```python
from build123d import *

# Parameters (mm, degrees)
F0_W     = 101.6
F0_H     = 101.6
F1_DEPTH = 9.525
F2_W     = 88.9
F2_H     = 88.9
F3_DEPTH = 3.175
F5_DEPTH = 3.175
F6_R     = 4.7625
F6_R_2   = 12.7
F7_DEPTH = 6.351
F8_R     = 3.175
F9_DEPTH = 9.526


with BuildPart() as f1:
    # F0 (on Top) → F1 (new body)
    with BuildSketch(Plane.XY):
        with Locations((50.8, 50.8)):
            Rectangle(F0_W, F0_H)
    extrude(amount=F1_DEPTH)

    # F2 (on face) → F3 (cut)
    with BuildSketch(Plane.XY.offset(9.525)):
        with Locations((50.8, 50.8)):
            Rectangle(F2_W, F2_H)
    extrude(amount=-F3_DEPTH, mode=Mode.SUBTRACT)

    # F4 (on face) → F5 (cut)
    with BuildSketch(Plane.XY.offset(9.525)):
        with BuildLine():
            Line((6.35, 95.25), (2.8575, 95.25))
            ThreePointArc((2.8575, 95.25), (1.2474604822, 94.8567465215), (0, 93.7655463142))
            Line((0, 93.7655463142), (0, 89.7494536858))
            ThreePointArc((0, 89.7494536858), (1.2474604822, 88.6582534785), (2.8575, 88.265))
            ThreePointArc((2.8575, 88.265), (5.3270704333, 87.2420704333), (6.35, 84.7725))
            Line((6.35, 84.7725), (6.35, 95.25))
        make_face()
        with BuildLine():
            ThreePointArc((2.8575, 13.335), (1.2474604822, 12.9417465215), (0, 11.8505463142))
            Line((0, 11.8505463142), (0, 7.8344536858))
            ThreePointArc((0, 7.8344536858), (1.2474604822, 6.7432534785), (2.8575, 6.35))
            Line((2.8575, 6.35), (6.35, 6.35))
            Line((6.35, 6.35), (6.35, 16.8275))
            ThreePointArc((6.35, 16.8275), (5.3270704333, 14.3579295667), (2.8575, 13.335))
        make_face()
        with BuildLine():
            ThreePointArc((98.7425, 13.335), (96.2729295667, 14.3579295667), (95.25, 16.8275))
            Line((95.25, 16.8275), (95.25, 6.35))
            Line((95.25, 6.35), (98.7425, 6.35))
            ThreePointArc((98.7425, 6.35), (100.3525395178, 6.7432534785), (101.6, 7.8344536858))
            Line((101.6, 7.8344536858), (101.6, 11.8505463142))
            ThreePointArc((101.6, 11.8505463142), (100.3525395178, 12.9417465215), (98.7425, 13.335))
        make_face()
        with BuildLine():
            Line((98.7425, 95.25), (95.25, 95.25))
            Line((95.25, 95.25), (95.25, 84.7725))
            ThreePointArc((95.25, 84.7725), (96.2729295667, 87.2420704333), (98.7425, 88.265))
            ThreePointArc((98.7425, 88.265), (100.3525395178, 88.6582534785), (101.6, 89.7494536858))
            Line((101.6, 89.7494536858), (101.6, 93.7655463142))
            ThreePointArc((101.6, 93.7655463142), (100.3525395178, 94.8567465215), (98.7425, 95.25))
        make_face()
    extrude(amount=-F5_DEPTH, mode=Mode.SUBTRACT)

    # F6 (on face) → F7 (cut, through all)
    with BuildSketch(Plane.XY.offset(6.35)):
        with Locations((23.8592316368, 77.7407683632)):
            Circle(F6_R)
        with Locations((77.7407683632, 77.7407683632)):
            Circle(F6_R)
        with Locations((77.7407683632, 23.8592316368)):
            Circle(F6_R)
        with Locations((23.8592316368, 23.8592316368)):
            Circle(F6_R)
        with Locations((50.8, 50.8)):
            Circle(F6_R_2)
    extrude(amount=-F7_DEPTH, mode=Mode.SUBTRACT)

    # F8 (on face) → F9 (cut, through all)
    with BuildSketch(Plane.XY.offset(9.525)):
        with Locations((12.7, 12.7)):
            Circle(F8_R)
        with Locations((88.9, 88.9)):
            Circle(F8_R)
        with Locations((12.7, 88.9)):
            Circle(F8_R)
        with Locations((88.9, 12.7)):
            Circle(F8_R)
    extrude(amount=-F9_DEPTH, mode=Mode.SUBTRACT)


solid = f1.part
```
Work out the finished part from the listing and answer in its coordinate system (mm). A direction names the side the tool comes from. Round coordinates to 2 decimals unless told otherwise and drop trailing zeros. Loops run counter-clockwise (first coordinate to the right, second up) from the corner with the lowest first, then second, coordinate; pieces in that order, holes last.
(1) The mould has two halves that part along Y. Classify faces 1 (the flat face through (50, 3, 9.525)), 2 (the flat face through (50, 101.6, 5)), 3 (the flat face through (51, 95.25, 8)): pulls with the +Y half, pulls with the -Y half, needs draft (parallel to the pull), parting line crosses it, or undercut.
Computed values:
face 1: needs draft
face 2: pulls with the +Y half
face 3: undercut
(2) The part is cut by section B-B, the plane y = 55.5. Give the vertices of the cut face in (x, z) (3 decimals).
Computed values:
outline: (0, 0) - (39.002, 0) - (39.002, 6.35) - (6.35, 6.35) - (6.35, 9.525) - (0, 9.525) - close; (62.598, 0) - (101.6, 0) - (101.6, 9.525) - (95.25, 9.525) - (95.25, 6.35) - (62.598, 6.35) - close
(3) The part is cut by section A-A, the plane x = 88.9. Give the vertices of the cut face in (y, z) (3 decimals), and give its area (3 significant figures).
Computed values:
outline: (0, 0) - (9.525, 0) - (9.525, 6.35) - (6.35, 6.35) - (6.35, 9.525) - (0, 9.525) - close; (15.875, 0) - (85.725, 0) - (85.725, 6.35) - (15.875, 6.35) - close; (92.075, 0) - (101.6, 0) - (101.6, 9.525) - (95.25, 9.525) - (95.25, 6.35) - (92.075, 6.35) - close
area: 605 mm2
(4) The part is cut by section C-C, the plane x = 55. Give the vertices of the cut face in (y, z) (3 decimals), and give its area (3 significant figures).
Computed values:
outline: (0, 0) - (38.815, 0) - (38.815, 6.35) - (6.35, 6.35) - (6.35, 9.525) - (0, 9.525) - close; (62.785, 0) - (101.6, 0) - (101.6, 9.525) - (95.25, 9.525) - (95.25, 6.35) - (62.785, 6.35) - close
area: 533 mm2
(5) Each of these flat-tipped pins is pushed along its axis until it touches: P1, Ø10, axis at x = 88.9, y = 12.7, coming from the -Z side; P2, Ø11, axis at x = 77.74, y = 23.86, coming from the +Z side. Where does it stop, or does it pass through?
Computed values:
P1: stops at z = 0
P2: stops at z = 6.35
(6) The part is cut by section D-D, the plane y = 81. Give the vertices of the cut face in (x, z) (3 decimals).
Computed values:
outline: (0, 0) - (20.387, 0) - (20.387, 6.35) - (6.35, 6.35) - (6.35, 9.525) - (0, 9.525) - close; (27.332, 0) - (74.268, 0) - (74.268, 6.35) - (27.332, 6.35) - close; (81.213, 0) - (101.6, 0) - (101.6, 9.525) - (95.25, 9.525) - (95.25, 6.35) - (81.213, 6.35) - close
(7) Find the intervals of material crossed by L1, parallel to Y at x = 88.9, z = 5.25 (3 decimals); L2, parallel to Y at x = 24.5, z = 0.5; L3, parallel to X at y = 82, z = 3.75, in increasing order.
Computed values:
L1: y = 0 to 9.525, 15.875 to 85.725, 92.075 to 101.6
L2: y = 0 to 19.14, 28.58 to 73.02, 82.46 to 101.6
L3: x = 0 to 21.73, 25.99 to 75.61, 79.87 to 101.6
(8) For faces 4 (the flat face through (6.35, 50, 8)), 5 (the flat face through (101.6, 50, 5)), determine the directions among +Z, -Z, +X, -X, +Y, -Y from which every point of the face is accessible in a straight line to the end or side of a thin tool.
Computed values:
face 4: +Z
face 5: +Z, -Z, +X, +Y, -Y
